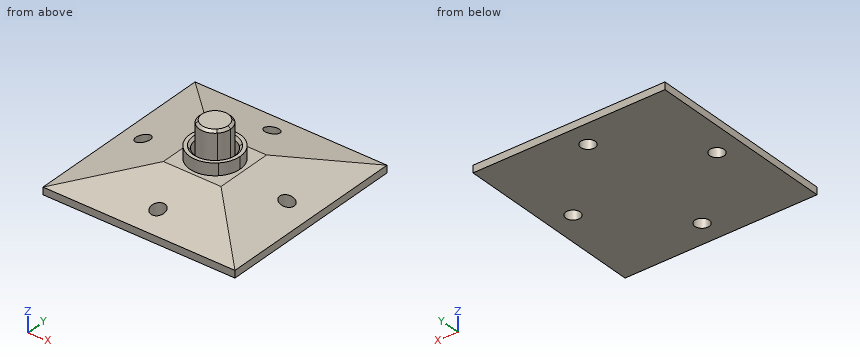
```python
from build123d import *

# Parameters (mm, degrees)
F0_R     = 3
F1_DEPTH = 10
F2_DEPTH = 15
F3_DEPTH = 5
F4_DEPTH = 25
F7_DEPTH = 80
F8_DEPTH = 80
F9_SIZE  = 1


with BuildPart() as f1:
    # F0 (on Top) → F1 (new body)
    with BuildSketch(Plane.XY):
        with BuildLine():
            ThreePointArc((-7.4246212025, 7.4246212025), (0, 10.5), (7.4246212025, 7.4246212025))
            Line((7.4246212025, 7.4246212025), (40, 40))
            Line((40, 40), (-40, 40))
            Line((-40, 40), (-7.4246212025, 7.4246212025))
        make_face()
        with Locations((0, 30)):
            Circle(F0_R, mode=Mode.SUBTRACT)
        with BuildLine():
            Line((40, 40), (7.4246212025, 7.4246212025))
            ThreePointArc((7.4246212025, 7.4246212025), (9.7007350914, 4.0181760398), (10.5, 0))
            ThreePointArc((10.5, 0), (9.7007350914, -4.0181760398), (7.4246212025, -7.4246212025))
            Line((7.4246212025, -7.4246212025), (40, -40))
            Line((40, -40), (40, 40))
        make_face()
        with Locations((30, 0)):
            Circle(F0_R, mode=Mode.SUBTRACT)
        with BuildLine():
            Line((40, -40), (7.4246212025, -7.4246212025))
            ThreePointArc((7.4246212025, -7.4246212025), (0, -10.5), (-7.4246212025, -7.4246212025))
            Line((-7.4246212025, -7.4246212025), (-40, -40))
            Line((-40, -40), (40, -40))
        make_face()
        with Locations((0, -30)):
            Circle(F0_R, mode=Mode.SUBTRACT)
        with BuildLine():
            ThreePointArc((-7.4246212025, -7.4246212025), (-10.5, 0), (-7.4246212025, 7.4246212025))
            Line((-7.4246212025, 7.4246212025), (-40, 40))
            Line((-40, 40), (-40, -40))
            Line((-40, -40), (-7.4246212025, -7.4246212025))
        make_face()
        with Locations((-30, 0)):
            Circle(F0_R, mode=Mode.SUBTRACT)
    extrude(amount=F1_DEPTH)

    # F0 (on Top) → F2 (join)
    with BuildSketch(Plane.XY):
        with BuildLine():
            ThreePointArc((-5.6568542495, 5.6568542495), (0, 8), (5.6568542495, 5.6568542495))
            Line((5.6568542495, 5.6568542495), (7.4246212025, 7.4246212025))
            ThreePointArc((7.4246212025, 7.4246212025), (0, 10.5), (-7.4246212025, 7.4246212025))
            Line((-7.4246212025, 7.4246212025), (-5.6568542495, 5.6568542495))
        make_face()
        with BuildLine():
            Line((7.4246212025, 7.4246212025), (5.6568542495, 5.6568542495))
            ThreePointArc((5.6568542495, 5.6568542495), (7.3910362601, 3.0614674589), (8, 0))
            ThreePointArc((8, 0), (7.3910362601, -3.0614674589), (5.6568542495, -5.6568542495))
            Line((5.6568542495, -5.6568542495), (7.4246212025, -7.4246212025))
            ThreePointArc((7.4246212025, -7.4246212025), (9.7007350914, -4.0181760398), (10.5, 0))
            ThreePointArc((10.5, 0), (9.7007350914, 4.0181760398), (7.4246212025, 7.4246212025))
        make_face()
        with BuildLine():
            Line((7.4246212025, -7.4246212025), (5.6568542495, -5.6568542495))
            ThreePointArc((5.6568542495, -5.6568542495), (0, -8), (-5.6568542495, -5.6568542495))
            Line((-5.6568542495, -5.6568542495), (-7.4246212025, -7.4246212025))
            ThreePointArc((-7.4246212025, -7.4246212025), (0, -10.5), (7.4246212025, -7.4246212025))
        make_face()
        with BuildLine():
            ThreePointArc((-5.6568542495, -5.6568542495), (-8, 0), (-5.6568542495, 5.6568542495))
            Line((-5.6568542495, 5.6568542495), (-7.4246212025, 7.4246212025))
            ThreePointArc((-7.4246212025, 7.4246212025), (-10.5, 0), (-7.4246212025, -7.4246212025))
            Line((-7.4246212025, -7.4246212025), (-5.6568542495, -5.6568542495))
        make_face()
    extrude(amount=F2_DEPTH)

    # F0 (on Top) → F3 (join)
    with BuildSketch(Plane.XY):
        with BuildLine():
            ThreePointArc((4.5961940777, 4.5961940777), (6.0052169613, 2.4874423104), (6.5, 0))
            ThreePointArc((6.5, 0), (6.0052169613, -2.4874423104), (4.5961940777, -4.5961940777))
            Line((4.5961940777, -4.5961940777), (5.6568542495, -5.6568542495))
            ThreePointArc((5.6568542495, -5.6568542495), (7.3910362601, -3.0614674589), (8, 0))
            ThreePointArc((8, 0), (7.3910362601, 3.0614674589), (5.6568542495, 5.6568542495))
            Line((5.6568542495, 5.6568542495), (4.5961940777, 4.5961940777))
        make_face()
        with BuildLine():
            Line((5.6568542495, -5.6568542495), (4.5961940777, -4.5961940777))
            ThreePointArc((4.5961940777, -4.5961940777), (0, -6.5), (-4.5961940777, -4.5961940777))
            Line((-4.5961940777, -4.5961940777), (-5.6568542495, -5.6568542495))
            ThreePointArc((-5.6568542495, -5.6568542495), (0, -8), (5.6568542495, -5.6568542495))
        make_face()
        with BuildLine():
            ThreePointArc((-4.5961940777, 4.5961940777), (0, 6.5), (4.5961940777, 4.5961940777))
            Line((4.5961940777, 4.5961940777), (5.6568542495, 5.6568542495))
            ThreePointArc((5.6568542495, 5.6568542495), (0, 8), (-5.6568542495, 5.6568542495))
            Line((-5.6568542495, 5.6568542495), (-4.5961940777, 4.5961940777))
        make_face()
        with BuildLine():
            ThreePointArc((-4.5961940777, -4.5961940777), (-6.5, 0), (-4.5961940777, 4.5961940777))
            Line((-4.5961940777, 4.5961940777), (-5.6568542495, 5.6568542495))
            ThreePointArc((-5.6568542495, 5.6568542495), (-8, 0), (-5.6568542495, -5.6568542495))
            Line((-5.6568542495, -5.6568542495), (-4.5961940777, -4.5961940777))
        make_face()
    extrude(amount=F3_DEPTH)

    # F0 (on Top) → F4 (join)
    with BuildSketch(Plane.XY):
        with BuildLine():
            ThreePointArc((4.5961940777, -4.5961940777), (6.0052169613, -2.4874423104), (6.5, 0))
            ThreePointArc((6.5, 0), (6.0052169613, 2.4874423104), (4.5961940777, 4.5961940777))
            Line((4.5961940777, 4.5961940777), (0, 0))
            Line((0, 0), (4.5961940777, -4.5961940777))
        make_face()
        with BuildLine():
            ThreePointArc((-4.5961940777, -4.5961940777), (0, -6.5), (4.5961940777, -4.5961940777))
            Line((4.5961940777, -4.5961940777), (0, 0))
            Line((0, 0), (-4.5961940777, -4.5961940777))
        make_face()
        with BuildLine():
            Line((0, 0), (-4.5961940777, 4.5961940777))
            ThreePointArc((-4.5961940777, 4.5961940777), (-6.5, 0), (-4.5961940777, -4.5961940777))
            Line((-4.5961940777, -4.5961940777), (0, 0))
        make_face()
        with BuildLine():
            Line((0, 0), (4.5961940777, 4.5961940777))
            ThreePointArc((4.5961940777, 4.5961940777), (0, 6.5), (-4.5961940777, 4.5961940777))
            Line((-4.5961940777, 4.5961940777), (0, 0))
        make_face()
    extrude(amount=F4_DEPTH)

    # F5 (on face) → F7 (cut)
    with BuildSketch(Plane.XZ.offset(40)):
        Polygon((-40, 3), (-12, 10), (-40, 10), align=None)
        Polygon((40, 10), (12, 10), (40, 3), align=None)
    extrude(amount=-F7_DEPTH, mode=Mode.SUBTRACT)

    # F6 (on face) → F8 (cut)
    with BuildSketch(Plane(origin=(-40, 0, 0), x_dir=(0, -1, 0), z_dir=(-1, 0, 0))):
        Polygon((-40, 3), (-12, 10), (-40, 10), align=None)
        Polygon((40, 10), (12, 10), (40, 3), align=None)
    extrude(amount=-F8_DEPTH, mode=Mode.SUBTRACT)

    # F9
    f9_edges = [f1.edges().sort_by_distance(p)[0] for p in [
        (5.656854, 5.656854, 15),
        (-4.596194, -4.596194, 25),
    ]]
    chamfer(f9_edges, length=F9_SIZE)


solid = f1.part
```
Input: part model. Units: mm. Frame: model coordinates. Coordinates: 2 decimals unless noted, no trailing zeros. Write each loop counter-clockwise with the first axis right and the second up, starting at its lowest first coordinate (ties: lowest second). Pieces come first, ordered by that corner, then holes.
1) Pin query (flat end, axial travel): pin 1 Ø6 at (y, z) = (3.5, 13.5) entering from -X; pin 2 Ø2 at (x, y) = (-21, -28.5) entering from -Z; pin 3 Ø8 at (x, y) = (0, -30) entering from +Z. Return the tip coordinate at first contact, or that it passes through.
2) Section D-D on x = -28.5. Output: boundary loops of the cut face in (y, z) (3 decimals), and give its area (3 significant figures).
3) Material intervals for line 1 along Y through (x, z) = (0, 1.5); line 2 along Y through (x, z) = (0, 5.25); line 3 along Y through (x, z) = (30, 1.75), sorted ascending.
4) Section B-B on x = 0. State how many separate pieces and enclosed holes the cut face has, and give its area (3 significant figures).
5) Section A-A on z = 11. Output: boundary loops of the cut face in (x, y), and give its area (3 significant figures).
6) Section C-C on y = 30. Output: boundary loops of the cut face in (x, z), and give its area (3 significant figures).
Check result:
1. pin 1: stops at x = -10.49
1. pin 2: stops at z = 0
1. pin 3: stops at z = 6.5
2. outline: (-40, 0) - (-2.598, 0) - (-2.598, 5.875) - (-28.5, 5.875) - (-40, 3) - close; (2.598, 0) - (40, 0) - (40, 3) - (28.5, 5.875) - (2.598, 5.875) - close
2. area: 406 mm2
3. line 1: y = -40 to -33, -27 to 27, 33 to 40
3. line 2: y = -27 to -8, -6.5 to 6.5, 8 to 27
3. line 3: y = -40 to -3, 3 to 40
4. separate pieces: 3
4. enclosed holes: 0
4. area: 741 mm2
5. outline: circle Ø21 at (0, 0); circle Ø13 at (0, 0); hole circle Ø16 at (0, 0)
5. area: 278 mm2
6. outline: (-40, 0) - (-3, 0) - (-3, 5.5) - (-30, 5.5) - (-40, 3) - close; (3, 0) - (40, 0) - (40, 3) - (30, 5.5) - (3, 5.5) - close
6. area: 382 mm2
